```python
from build123d import *

# Parameters (mm, degrees)
F0_W     = 12
F0_H     = 12
F1_DEPTH = 75
F3_DEPTH = 10
F4_SIZE  = 0.3


# Not quite as in the source:
# - a pattern or mirror of a feature is missing from the dataset's text; its kind, count and spacing are read off the source's solid


with BuildPart() as f1:
    # F0 (on Top) → F1 (new body, symmetric)
    with BuildSketch(Plane.XY):
        Rectangle(F0_W, F0_H)
    extrude(amount=F1_DEPTH, both=True)

    # F2 (on face) → F3 (join)
    with BuildSketch(Plane.XY.offset(75)):
        Polygon((-0.3250005729, 4), (-4, 4), (-4, 0.325), (-4, -0.325), (-4, -4), (-0.3250005729, -4), (0.3250005729, -4), (4, -4), (4, -0.325), (4, 0.325), (4, 4), (0.3250005729, 4), align=None)
        with BuildLine():
            ThreePointArc((0.3250005729, 4), (0, 4.3250005729), (-0.3250005729, 4))
            Line((-0.3250005729, 4), (0.3250005729, 4))
        make_face()
        with BuildLine():
            Line((-4, -0.325), (-4, 0.325))
            ThreePointArc((-4, 0.325), (-4.325, 0), (-4, -0.325))
        make_face()
        with BuildLine():
            ThreePointArc((4, -0.325), (4.325, 0), (4, 0.325))
            Line((4, 0.325), (4, -0.325))
        make_face()
        with BuildLine():
            Line((0.3250005729, -4), (-0.3250005729, -4))
            ThreePointArc((-0.3250005729, -4), (0, -4.3250005729), (0.3250005729, -4))
        make_face()
    f3 = extrude(amount=F3_DEPTH)

    # F3_copies: F3 across plane
    add(f3.mirror(Plane(origin=(0, 0, 0), x_dir=(-1, 0, 0), z_dir=(0, 0, -1))))

    # F4
    f4_edges = [f1.edges().sort_by_distance(p)[0] for p in [
        (0, -4.325001, 85),
        (4.325, 0, 85),
        (0, 4.325001, 85),
        (-4.325, 0, 85),
        (-4.325, 0, -85),
        (0, -4.325001, -85),
        (4.325, 0, -85),
        (0, 4.325001, -85),
    ]]
    chamfer(f4_edges, length=F4_SIZE)


solid = f1.part
```
Work out the finished part from the listing and answer in its coordinate system (mm). A direction names the side the tool comes from. Give positions to 0.01 mm unless a question says otherwise; leave off trailing zeros. Order: outer loops, then holes, each group sorted by start corner. A loop starts at its lowest first (then second) coordinate and runs counter-clockwise, first axis right, second up.
1. A straight line is drawn through the part: L1, parallel to Z at x = 1.75, y = -5. Find the intervals that lie inside material, in ascending order.
Result sheet:
L1: z = -75 to 75
2. Section A-A, the plane y = 1.75 is taken. Determine the outline of the cut face in (x, z).
Result sheet:
outline: (-6, -75) - (-4, -75) - (-4, -85) - (4, -85) - (4, -75) - (6, -75) - (6, 75) - (4, 75) - (4, 85) - (-4, 85) - (-4, 75) - (-6, 75) - close
3. Each of these flat-tipped pins is pushed along its axis until it touches: P1, Ø4.5, axis at y = -1, z = -79.5, coming from the +X side (3 decimals); P2, Ø3, axis at x = 1.5, z = -79.5, coming from the +Y side (3 decimals); P3, Ø1.2, axis at y = 1, z = -81.5, coming from the +X side. Where does it stop, or does it pass through?
Result sheet:
P1: stops at x = 4.325
P2: stops at y = 4.325
P3: stops at x = 4
4. For faces 1 (the flat face through (4, -2, -80)), 2 (the flat face through (-2, 4, -80)), 3 (the flat face through (4, 2, -80)), 4 (the flat face through (4, -2, 80)), 5 (the flat face through (-4, -2, -80)), determine the directions among +Z, -Z, +X, -X, +Y, -Y from which every point of the face is accessible in a straight line to the end or side of a thin tool.
Result sheet:
face 1: -Z, +X, -Y
face 2: -Z, -X, +Y
face 3: -Z, +X, +Y
face 4: +Z, +X, -Y
face 5: -Z, -X, -Y
